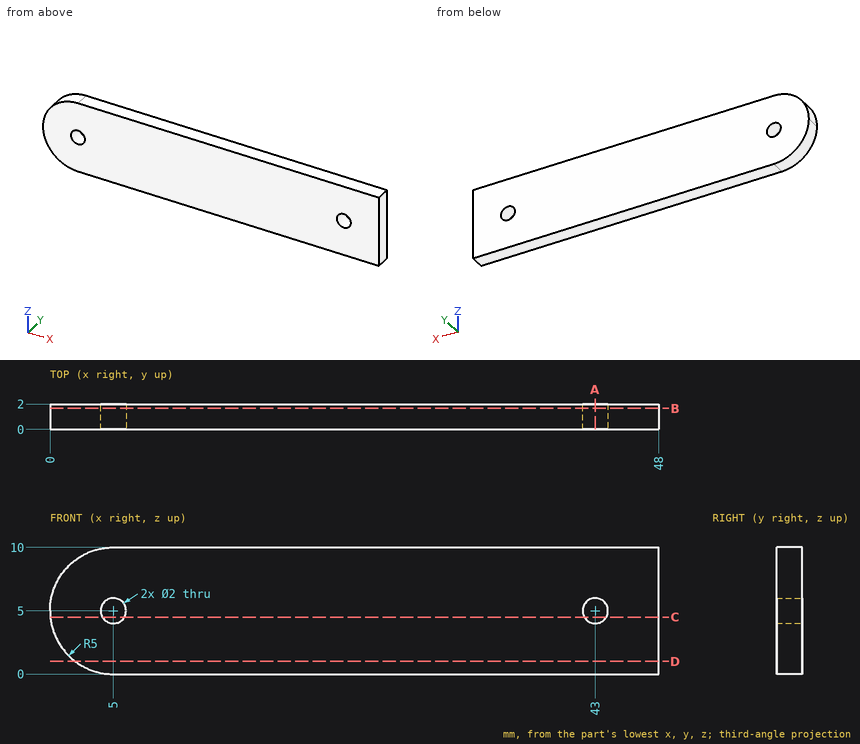
Can you work these out from the drawing? Everything is in mm from the part's minimum corner. Round coordinates to 2 decimals unless told otherwise and drop trailing zeros. Write each loop counter-clockwise with the first axis right and the second up, starting at its lowest first coordinate (ties: lowest second). Pieces come first, ordered by that corner, then holes. Notation, with made-up numbers: (29.25, -29) - (58.25, -29) arc R14 cw to (58.25, -17) - close; hole circle Ø1 at (-8.5, 58.5). An arc over 180 degrees is marked (long way). Use a Markdown table: item, result.
Q1. Please list where these lines run through material, in increasing order: L1, parallel to Z at x = 5, y = 1.45; L2, parallel to X at y = 0.35, z = 4.75; L3, parallel to X at y = 1.4, z = 1.75.
Output values:
| item | result |
|---|---|
| L1 | 0 to 4, 6 to 10 |
| L2 | 0.01 to 4.03, 5.97 to 42.03, 43.97 to 48 |
| L3 | 1.2 to 48 |
Q2. I want a section at D-D (z = 1). List the corners of the cut face in (x, y) for me.
Output values:
| item | result |
|---|---|
| outline | (2, 0) - (48, 0) - (48, 2) - (2, 2) - close |
Q3. I want a section at C-C (z = 4.5). List the corners of the cut face in (x, y) for me.
Output values:
| item | result |
|---|---|
| outline | (0.03, 0) - (4.13, 0) - (4.13, 2) - (0.03, 2) - close; (5.87, 0) - (42.13, 0) - (42.13, 2) - (5.87, 2) - close; (43.87, 0) - (48, 0) - (48, 2) - (43.87, 2) - close |
Q4. For pin 1 (3 mm diameter, centred on x = 43, z = 5, fed in from +Y), with a flat end and sliding along its axis, tell me the tip position at first contact or that it passes through.
Output values:
| item | result |
|---|---|
| pin 1 | y = 2 |
Q5. I want a section at A-A (x = 43). List the corners of the cut face in (y, z) for me.
Output values:
| item | result |
|---|---|
| outline | (0, 0) - (2, 0) - (2, 4) - (0, 4) - close; (0, 6) - (2, 6) - (2, 10) - (0, 10) - close |
Q6. I want a section at B-B (y = 1.65). Count the separate pieces of the cut face and the enclosed holes in it, plus the area to 3 significant figures.
Output values:
| item | result |
|---|---|
| separate pieces | 1 |
| enclosed holes | 2 |
| area | 463 mm2 |
